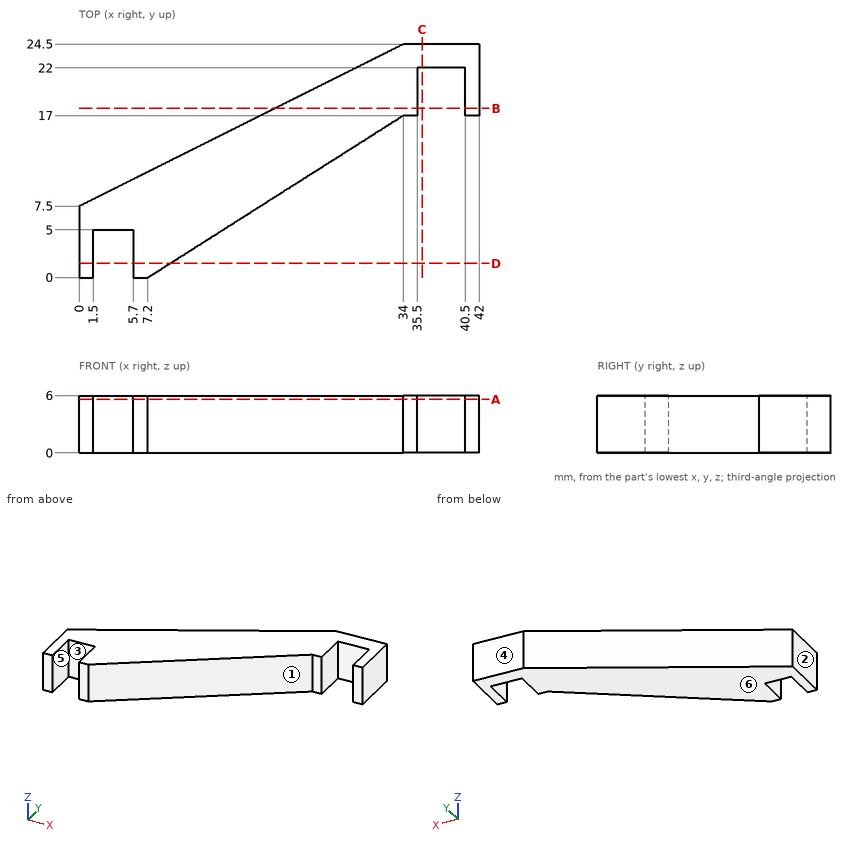
Job drawing, mm, ordinate dimensions from the low corner. One solid piece. A direction names the side the tool comes from. Give positions to 0.01 mm unless a question says otherwise; leave off trailing zeros. Loops run counter-clockwise (first coordinate to the right, second up) from the corner with the lowest first, then second, coordinate; pieces in that order, holes last. Notation, with made-up numbers: M 26.25,20.25 L 43.25,20.25 A12 ccw 43.25,42.25 Z; hole C 30.25,-3.75 d3. An arc over 180 degrees is marked long. Put each result on its own line as item: value. Start each with the question number.
1) Flat gauge pins, fed straight in: pin 1 (2 mm diameter, centred on x = 4, z = 2.5, fed in from -Y); pin 2 (3 mm diameter, centred on x = 17, y = 2.5, fed in from +Z); pin 3 (1.6 mm diameter, centred on x = 34.5, z = 3.5, fed in from -Y); pin 4 (2.5 mm diameter, centred on y = 1.5, z = 3.5, fed in from -X). Where does each tip first touch, or does it go through?
2) Saw through at A-A (z = 5.6). List the corners of the cut face in (x, y), then the cut area to 3 significant figures.
3) Saw through at B-B (y = 17.75). List the corners of the cut face in (x, z), then the cut area to 3 significant figures.
4) Probe probe 1 along Y at (x, z) = (35, 2.95); probe 2 along X at (y, z) = (21.25, 2.6); probe 3 along X at (y, z) = (18.25, 4.55). List the from-to ranges inside material, lowest first.
5) Saw through at C-C (x = 36). List the corners of the cut face in (y, z), then the cut area to 3 significant figures.
6) Pull direction X, two halves, no side cores. Call the marked faces 1, 2, 3 and 4: +X half, -X half, draft (parallel to the pull), parting line (faces both ways), or undercut.
7) 3-axis set-ups, long thin cutter, end or side, ignore diameter. For the marked faces 5 and 6: which of +Z, -Z, +X, -X, +Y, -Y reach the whole face in a straight line?
8) Saw through at D-D (y = 1.5). List the corners of the cut face in (x, z).
Numbers:
1. pin 1: y = 5
1. pin 2: through
1. pin 3: y = 16.81
1. pin 4: x = 0
2. outline: M 0,0 L 1.5,0 L 1.5,5 L 5.7,5 L 5.7,0 L 7.2,0 L 34,17 L 35.5,17 L 35.5,22 L 40.5,22 L 40.5,17 L 42,17 L 42,24.5 L 34,24.5 L 0,7.5 Z
2. area: 330 mm^2
3. outline: M 20.5,0 L 35.5,0 L 35.5,6 L 20.5,6 Z; M 40.5,0 L 42,0 L 42,6 L 40.5,6 Z
3. area: 99.0 mm^2
4. probe 1: 17 to 24.5
4. probe 2: 27.5 to 35.5, 40.5 to 42
4. probe 3: 21.5 to 35.5, 40.5 to 42
5. outline: M 22,0 L 24.5,0 L 24.5,6 L 22,6 Z
5. area: 15.0 mm^2
6. face 1: +X half
6. face 2: -X half
6. face 3: undercut
6. face 4: draft
7. face 5: +Z, -Z, -Y
7. face 6: -Z, +X, -X, +Y, -Y
8. outline: M 0,0 L 1.5,0 L 1.5,6 L 0,6 Z; M 5.7,0 L 9.56,0 L 9.56,6 L 5.7,6 Z
